```python
from build123d import *

# Parameters (mm, degrees)
SKETCH_1_W       = 15
SKETCH_1_H       = 32
EXTRUDE_1_DEPTH  = 1
SKETCH_2_W       = 1
SKETCH_2_H       = 32
EXTRUDE_2_DEPTH  = 20
SKETCH_8_W       = 32
SKETCH_8_H       = 1
EXTRUDE_8_DEPTH  = 15
SKETCH_9_W       = 13.087276504
SKETCH_9_H       = 20
EXTRUDE_9_DEPTH  = 15
SKETCH_10_R      = 2.796797866
EXTRUDE_10_DEPTH = 3


with BuildPart() as part:
    # 草图1 → 凸台-拉伸1 (new body)
    with BuildSketch(Plane(origin=(0, 0, 0), x_dir=(1, 0, 0), z_dir=(0, 1, 0))):
        Rectangle(SKETCH_1_W, SKETCH_1_H)
    extrude(amount=EXTRUDE_1_DEPTH)

    # 草图2 → 凸台-拉伸2 (add)
    with BuildSketch(Plane(origin=(0, 1, 0), x_dir=(1, 0, 0), z_dir=(0, 1, 0))):
        with Locations((-7, 0)):
            Rectangle(SKETCH_2_W, SKETCH_2_H)
    extrude(amount=EXTRUDE_2_DEPTH)

    # 草图8 → 凸台-拉伸8 (add)
    with BuildSketch(Plane.ZY.offset(7.5)):
        with Locations((0, 20.5)):
            Rectangle(SKETCH_8_W, SKETCH_8_H)
    extrude(amount=EXTRUDE_8_DEPTH)

    # 草图9 → 凸台-拉伸9 (add)
    with BuildSketch(Plane(origin=(0, 21, 0), x_dir=(1, 0, 0), z_dir=(0, 1, 0))):
        with Locations((-14.334681212, 0.503703775)):
            Rectangle(SKETCH_9_W, SKETCH_9_H)
    extrude(amount=EXTRUDE_9_DEPTH)

    # 草图10 → 凸台-拉伸10 (add)
    with BuildSketch(Plane.ZY.offset(20.878319464)):
        with Locations(Location((0, 28.5, 0), (0, 0, 180))):
            Circle(SKETCH_10_R)
    extrude(amount=EXTRUDE_10_DEPTH)


solid = part.part
```
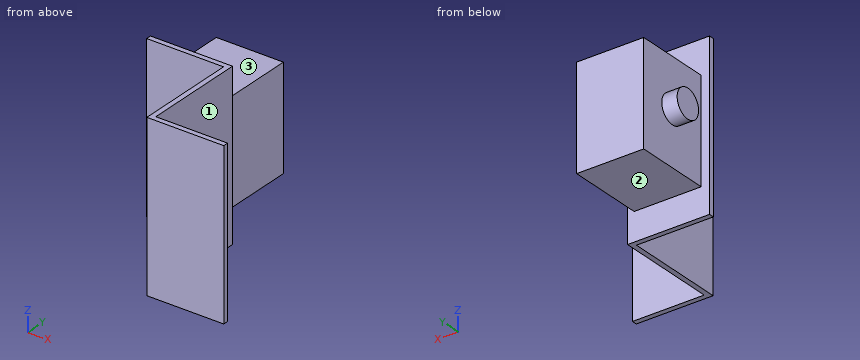
Geometry check sheet. Reference: the model listing, model coordinates, mm. Face numbers are marked on the shaded views. A direction names the side the tool comes from. Give positions to 0.01 mm unless a question says otherwise; leave off trailing zeros. Loops run counter-clockwise (first coordinate to the right, second up) from the corner with the lowest first, then second, coordinate; pieces in that order, holes last. Notation, with made-up numbers: (20.25, 76.5) - (43.25, 76.5) arc R12 ccw to (43.25, 82.5) - close; hole circle Ø7 at (10.25, 47.25). An arc over 180 degrees is marked (long way). Use CSV: the item, a comma, the result in double quotes. Start each with the question number.
Q1. Access from +Z, -Z, +X, -X, +Y, -Y to the whole of each face (thin tool, end or side, straight path). Record for the marked faces 1, 2 and 3.
Q2. Section check B-B, the plane y = 28.5. Record the cut outline in (x, z).
Q3. Section check D-D, the plane z = 0. Record the cut outline in (x, y).
Q4. Section check C-C, the plane x = -13. Record the cut outline in (y, z), and give its area (3 significant figures).
Q5. Scan lines: probe 1 along Y at (x, z) = (0.5, 5.5); probe 2 along Y at (x, z) = (-11, -11.5); probe 3 along X at (y, z) = (17, 7). Record each from-to range of solid material in increasing order. Write a range as from..to.
Q6. Section check A-A, the plane z = -6.5. Record the cut outline in (x, y), and give its area (3 significant figures).
Q7. Go/stop test with flat-tipped pins: pin 1 Ø10 at (y, z) = (11.5, -7) entering from +X; pin 2 Ø1 at (y, z) = (22, -6.5) entering from +X; pin 3 Ø6.5 at (x, y) = (-17.5, 31) entering from -Z; pin 4 Ø6 at (x, y) = (-1.5, 9.5) entering from -Z. Record where each tip stops, or that it passes through.
Findings below:
1,face 1,"+Z, -Z, +X, +Y"
1,face 2,"-Z, +X, -X, +Y"
1,face 3,"+Z, +X, -X, +Y"
2,outline,"(-23.88, -2.8) - (-20.88, -2.8) - (-20.88, -10.5) - (-7.79, -10.5) - (-7.79, 9.5) - (-20.88, 9.5) - (-20.88, 2.8) - (-23.88, 2.8) - close"
3,outline,"(-23.88, 25.7) - (-20.88, 25.7) - (-20.88, 21) - (-22.5, 21) - (-22.5, 20) - (-7.5, 20) - (-7.5, 0) - (7.5, 0) - (7.5, 1) - (-6.5, 1) - (-6.5, 21) - (-7.79, 21) - (-7.79, 36) - (-20.88, 36) - (-20.88, 31.3) - (-23.88, 31.3) - close"
4,outline,"(20, -16) - (21, -16) - (21, -10.5) - (36, -10.5) - (36, 9.5) - (21, 9.5) - (21, 16) - (20, 16) - close"
4,area,"332 mm^2"
5,probe 1,"y = 0..1"
5,probe 2,"y = 20..21"
5,probe 3,"x = -7.5..-6.5"
6,outline,"(-22.5, 20) - (-7.5, 20) - (-7.5, 0) - (7.5, 0) - (7.5, 1) - (-6.5, 1) - (-6.5, 21) - (-7.79, 21) - (-7.79, 36) - (-20.88, 36) - (-20.88, 21) - (-22.5, 21) - close"
6,area,"246 mm^2"
7,pin 1,"stops at x = -6.5"
7,pin 2,"stops at x = -7.79"
7,pin 3,"stops at z = -10.5"
7,pin 4,"passes through"
